Source: CAD feature listing. Evaluate the final solid. Frame: model axes, mm. Face numbers are marked on the shaded views. Give positions to 0.01 mm unless a question says otherwise; leave off trailing zeros. Loops run counter-clockwise (first coordinate to the right, second up) from the corner with the lowest first, then second, coordinate; pieces in that order, holes last. Notation, with made-up numbers: M -39,-22.75 L 20,-22.75 A21 cw 20,-9.75 Z; hole C 87,55 d6. An arc over 180 degrees is marked long. Answer in a Markdown table with one row per item.
```python
from build123d import *

# Parameters (mm, degrees)
F0_W     = 49
F0_H     = 71.6
F0_W_2   = 46.3
F0_H_2   = 68.9
F1_DEPTH = 4
F2_DEPTH = 2
F3_W     = 5.65
F3_H     = 10
F3_R     = 1.5
F3_W_2   = 1.35
F4_DEPTH = 1
F5_DEPTH = 4.9


with BuildPart() as f1:
    # F0 (on Top) → F1 (new body)
    with BuildSketch(Plane.XY):
        Rectangle(F0_W, F0_H)
        Rectangle(F0_W_2, F0_H_2, mode=Mode.SUBTRACT)
    extrude(amount=F1_DEPTH)

    # F0 (on Top) → F2 (join)
    with BuildSketch(Plane.XY):
        Rectangle(F0_W_2, F0_H_2)
    extrude(amount=F2_DEPTH)

    # F3 (on face) → F4 (cut)
    with BuildSketch(Plane.XY):
        with Locations((-20.325, 0)):
            Rectangle(F3_W, F3_H)
        with Locations((-21, 0)):
            Circle(F3_R, mode=Mode.SUBTRACT)
        with Locations((-23.825, 0)):
            Rectangle(F3_W_2, F3_H)
    extrude(amount=F4_DEPTH, mode=Mode.SUBTRACT)

    # F3 (on face) → F5 (cut)
    with BuildSketch(Plane.XY):
        with Locations((-21, 0)):
            Circle(F3_R)
    extrude(amount=F5_DEPTH, mode=Mode.SUBTRACT)


solid = f1.part
```
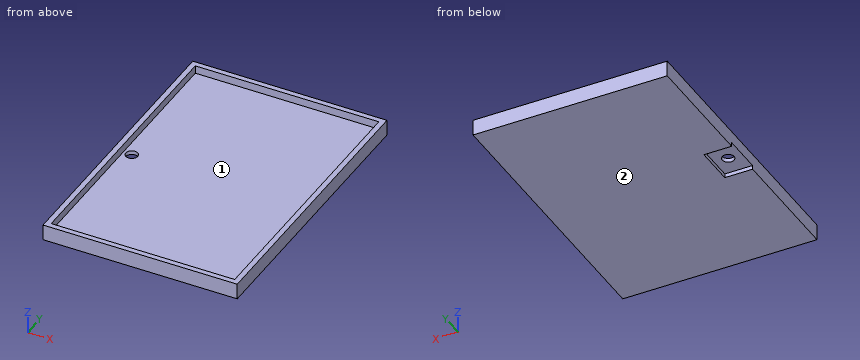
1) Section A-A, the plane y = 0. Return loops of the section in (x, z).
Reply:
| item | result |
|---|---|
| outline | M -24.5,1 L -22.5,1 L -22.5,2 L -23.15,2 L -23.15,4 L -24.5,4 Z; M -19.5,1 L -17.5,1 L -17.5,0 L 24.5,0 L 24.5,4 L 23.15,4 L 23.15,2 L -19.5,2 Z |
2) Section C-C, the plane y = -22. Return loops of the section in (x, z).
Reply:
| item | result |
|---|---|
| outline | M -24.5,0 L 24.5,0 L 24.5,4 L 23.15,4 L 23.15,2 L -23.15,2 L -23.15,4 L -24.5,4 Z |
3) Material intervals for L1, parallel to Y at x = -17.5, z = 2.5; L2, parallel to X at y = -31.5, z = 3.8; L3, parallel to Y at x = -21, z = 1.4, sorted ascending.
Reply:
| item | result |
|---|---|
| L1 | y = -35.8 to -34.45, 34.45 to 35.8 |
| L2 | x = -24.5 to -23.15, 23.15 to 24.5 |
| L3 | y = -35.8 to -1.5, 1.5 to 35.8 |
4) Section B-B, the plane x = -21. Return loops of the section in (y, z), then the cut area to 3 significant figures.
Reply:
| item | result |
|---|---|
| outline | M -35.8,0 L -5,0 L -5,1 L -1.5,1 L -1.5,2 L -34.45,2 L -34.45,4 L -35.8,4 Z; M 1.5,1 L 5,1 L 5,0 L 35.8,0 L 35.8,4 L 34.45,4 L 34.45,2 L 1.5,2 Z |
| area | 136 mm² |
5) Pull-direction query (Y, two-part tool) for the marked faces 1 and 2; classes: released by +Y, released by -Y, zero draft, split by the parting line, or undercut.
Reply:
| item | result |
|---|---|
| face 1 | undercut |
| face 2 | zero draft |
6) Pin query (flat end, axial travel): pin 1 Ø5 at (x, y) = (-21, 0) entering from -Z; pin 2 Ø23 at (x, y) = (-10.5, -0.5) entering from +Z; pin 3 Ø12 at (x, y) = (-12, 26) entering from -Z. Return the tip coordinate at first contact, or that it passes through.
Reply:
| item | result |
|---|---|
| pin 1 | stops at z = 1 |
| pin 2 | stops at z = 2 |
| pin 3 | stops at z = 0 |
7) Section D-D, the plane x = -14.5. Return loops of the section in (y, z).
Reply:
| item | result |
|---|---|
| outline | M -35.8,0 L 35.8,0 L 35.8,4 L 34.45,4 L 34.45,2 L -34.45,2 L -34.45,4 L -35.8,4 Z |
